```python
from build123d import *

# Parameters (mm, degrees)
SKETCH050_W       = 15
SKETCH050_H       = 9
SKETCH050_R       = 1.7
PAD025_DEPTH      = 17
BOX002_W          = 6
BOX002_H          = 10
BOX002_DEPTH      = 2.8
BOX003_W          = 17
BOX003_H          = 10
BOX003_DEPTH      = 12
CYLINDER002_R     = 1.7
CYLINDER002_DEPTH = 10
CYLINDER003_R     = 1.7
CYLINDER003_DEPTH = 10


with BuildPart() as part:
    # Sketch050 → Pad025 (new body)
    with BuildSketch(Plane.XY):
        Rectangle(SKETCH050_W, SKETCH050_H)
        Circle(SKETCH050_R, mode=Mode.SUBTRACT)
    extrude(amount=PAD025_DEPTH)

    # Box002 → Box002 (cut)
    with BuildSketch(Plane(origin=(-3, -6.5, 12), x_dir=(1, 0, 0), z_dir=(0, 0, 1))):
        with Locations((3, 5)):
            Rectangle(BOX002_W, BOX002_H)
    extrude(amount=BOX002_DEPTH, mode=Mode.SUBTRACT)

    # Box003 → Box003 (cut)
    with BuildSketch(Plane(origin=(-8, -8, -2), x_dir=(1, 0, 0), z_dir=(0, 0, 1))):
        with Locations((8.5, 5)):
            Rectangle(BOX003_W, BOX003_H)
    extrude(amount=BOX003_DEPTH, mode=Mode.SUBTRACT)

    # Cylinder002 → Cylinder002 (cut)
    with BuildSketch(Plane(origin=(-4, 7, 5), x_dir=(1, 0, 0), z_dir=(0, -1, 0))):
        Circle(CYLINDER002_R)
    extrude(amount=CYLINDER002_DEPTH, mode=Mode.SUBTRACT)

    # Cylinder003 → Cylinder003 (cut)
    with BuildSketch(Plane(origin=(4, 7, 5), x_dir=(1, 0, 0), z_dir=(0, -1, 0))):
        Circle(CYLINDER003_R)
    extrude(amount=CYLINDER003_DEPTH, mode=Mode.SUBTRACT)


solid = part.part
```
Work out the finished part from the listing and answer in its coordinate system (mm). A direction names the side the tool comes from. Coordinates: 2 decimals unless noted, no trailing zeros. Write each loop counter-clockwise with the first axis right and the second up, starting at its lowest first coordinate (ties: lowest second). Pieces come first, ordered by that corner, then holes. Notation, with made-up numbers: (13.25, 50.25) - (42.25, 50.25) arc R31 ccw to (42.25, 88.25) - close; hole circle Ø11 at (28.5, 87.5). An arc over 180 degrees is marked (long way). Answer as a JSON object with one key per item and string values.
Q1. Find section A-A (y = 0). Write down the section's boundary in (x, z), plus the area to 3 significant figures.
Results list:
{"outline": "(-7.5, 10) - (-1.7, 10) - (-1.7, 12) - (-3, 12) - (-3, 14.8) - (-1.7, 14.8) - (-1.7, 17) - (-7.5, 17) - close; (1.7, 10) - (7.5, 10) - (7.5, 17) - (1.7, 17) - (1.7, 14.8) - (3, 14.8) - (3, 12) - (1.7, 12) - close", "area": "73.9 mm^2"}
Q2. Which of the six approach directions +Z, -Z, +X, -X, +Y, -Y give full straight-line access (tool end or side, diameter ignored) to faces 4 (the flat face through (-7.5, 1, 12)), 5 (the flat face through (0, 3.5, 13)), 6 (the flat face through (0, -2, 10))?
Results list:
{"face 4": "+Z, -Z, -X, +Y, -Y", "face 5": "-Y", "face 6": "-Z, +X, -X, -Y"}
Q3. Given pin 1 Ø5 at (x, y) = (1.5, 0) entering from -Z; pin 2 Ø1.4 at (x, z) = (-0.5, 13) entering from -Y; pin 3 Ø5 at (x, z) = (3, 3) entering from -Y; pin 4 Ø2 at (x, y) = (-0.5, -1) entering from -Z, each flat-ended and moving along its own axis, determine where each tip first touches the part or whether it passes through.
Results list:
{"pin 1": "stops at z = 0", "pin 2": "stops at y = 3.5", "pin 3": "stops at y = 2", "pin 4": "stops at z = 10"}
Q4. Consider L1, parallel to X at y = 2.65, z = 5; L2, parallel to Z at x = 1.5, y = 1.5; L3, parallel to Z at x = -4, y = 3.2. Determine where each line is inside the solid, lowest interval first. Write a range as from..to.
Results list:
{"L1": "x = -7.5..-5.7, -2.3..2.3, 5.7..7.5", "L2": "z = 10..12, 14.8..17", "L3": "z = 0..3.3, 6.7..17"}
Q5. Find section B-B (x = -4). Write down the section's boundary in (y, z).
Results list:
{"outline": "(-4.5, 10) - (2, 10) - (2, 6.7) - (4.5, 6.7) - (4.5, 17) - (-4.5, 17) - close; (2, 0) - (4.5, 0) - (4.5, 3.3) - (2, 3.3) - close"}
Q6. Find section C-C (y = 4). Write down the section's boundary in (x, z), plus the area to 3 significant figures.
Results list:
{"outline": "(-7.5, 0) - (7.5, 0) - (7.5, 17) - (-7.5, 17) - close; hole circle Ø3.4 at (-4, 5); hole circle Ø3.4 at (4, 5)", "area": "237 mm^2"}
Q7. For a pull along X with two mould halves and no side action, classify faces 1 (the flat face through (7.5, 1, 12)), 2 (the flat face through (0, 2, 5)), 3 (the flat face through (1.29, -1.33, 14.8)) as pulls with the +X half, pulls with the -X half, needs draft (parallel to the pull), parting line crosses it, or undercut.
Results list:
{"face 1": "pulls with the +X half", "face 2": "needs draft", "face 3": "undercut"}
Q8. Find section D-D (x = 0). Write down the section's boundary in (y, z), plus the area to 3 significant figures.
Results list:
{"outline": "(-4.5, 10) - (-1.7, 10) - (-1.7, 12) - (-4.5, 12) - close; (-4.5, 14.8) - (-1.7, 14.8) - (-1.7, 17) - (-4.5, 17) - close; (1.7, 10) - (2, 10) - (2, 0) - (4.5, 0) - (4.5, 17) - (1.7, 17) - (1.7, 14.8) - (3.5, 14.8) - (3.5, 12) - (1.7, 12) - close", "area": "51.3 mm^2"}
